The model under review builds one solid part; all positions refer to its coordinate system, in mm. Face numbers are marked on the shaded views. Give positions to 0.01 mm unless a question says otherwise; leave off trailing zeros. Loops run counter-clockwise (first coordinate to the right, second up) from the corner with the lowest first, then second, coordinate; pieces in that order, holes last. Notation, with made-up numbers: M -23.75,84 L 8.25,84 A14 cw 8.25,92 Z; hole C 5,58.25 d4. An arc over 180 degrees is marked long. Return JSON: item names as keys, results as strings. Group by question number.
```python
from build123d import *

# Parameters (mm, degrees)
F0_W     = 85
F0_H     = 19.05
F1_DEPTH = 6.35
F2_R     = 3
F3_R     = 1.535965
F3_R_2   = 4.709265
F4_DEPTH = 25
F5_R     = 1.5
F6_DEPTH = 5


with BuildPart() as f1:
    # F0 (on Front) → F1 (new body)
    with BuildSketch(Plane.XZ):
        Rectangle(F0_W, F0_H)
    extrude(amount=F1_DEPTH)

    # F2
    f2_edges = [f1.edges().sort_by_distance(p)[0] for p in [
        (-42.5, -3.175, 9.525),
        (42.5, -3.175, 9.525),
        (-42.5, -3.175, -9.525),
        (42.5, -3.175, -9.525),
    ]]
    fillet(f2_edges, radius=F2_R)

    # F3 (on face) → F4 (cut)
    with BuildSketch(Plane.XZ.offset(6.35)):
        with Locations((-19.519491, 0)):
            Circle(F3_R)
        with Locations((27.747195, 0)):
            Circle(F3_R_2)
    extrude(amount=-F4_DEPTH, mode=Mode.SUBTRACT)

    # F5 (on face) → F6 (cut)
    with BuildSketch(Plane(origin=(0, 0, -9.525), x_dir=(1, 0, 0), z_dir=(0, 0, -1))):
        with Locations((-21, 3.0625)):
            Circle(F5_R)
        with Locations((21.000085, 3.118848)):
            Circle(F5_R)
    extrude(amount=-F6_DEPTH, mode=Mode.SUBTRACT)


solid = f1.part
```
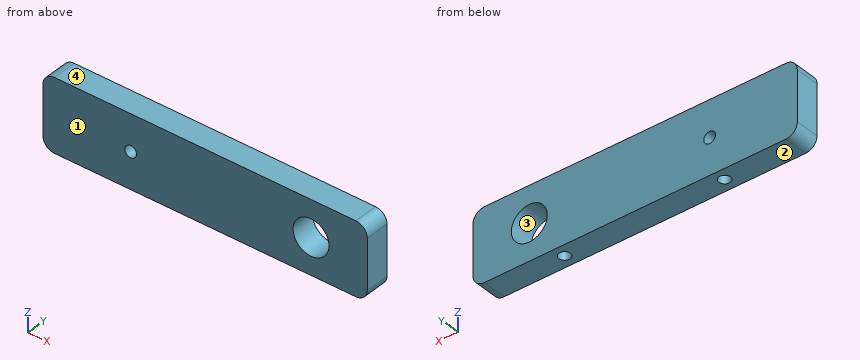
(1) Add section B-B (z = 3.5). Write out the cut boundary in (x, y), and give its area (3 significant figures).
(2) Add section C-C (x = 27). Write out the cut boundary in (y, z) (3 decimals).
(3) Add section A-A (z = 0). Write out the cut boundary in (x, y).
(4) Mouldability with a two-part tool opening along Z and no side actions: class the marked faces 1, 2, 3 and 4 as released by +Z, released by -Z, zero draft, split by the parting line, or undercut.
(5) Add section D-D (z = -8). Write out the cut boundary in (x, y), and give its area (3 significant figures).
(6) For probe 1 along X at (y, z) = (-3.5, 0.5); probe 2 along X at (y, z) = (-3.5, -1); probe 3 along X at (y, z) = (-1.75, -3.5), list the stretches that pass through material, from the lowest coordinate up.
(7) For pin 1 (6 mm diameter, centred on x = -25, z = -3, fed in from +Y); pin 2 (1.5 mm diameter, centred on x = 21.5, y = -3, fed in from -Z) (3 decimals); pin 3 (2.5 mm diameter, centred on x = -19.52, z = 0, fed in from +Y), all flat-tipped, find the tip position at first contact; note any pin that passes through.
Verdict:
{
 "1": {"outline": "M -42.5,-6.35 L 24.6,-6.35 L 24.6,0 L -42.5,0 Z; M 30.9,-6.35 L 42.5,-6.35 L 42.5,0 L 30.9,0 Z", "area": "500 mm²"},
 "2": {"outline": "M -6.35,-9.525 L 0,-9.525 L 0,-4.65 L -6.35,-4.65 Z; M -6.35,4.65 L 0,4.65 L 0,9.525 L -6.35,9.525 Z"},
 "3": {"outline": "M -42.5,-6.35 L -21.06,-6.35 L -21.06,0 L -42.5,0 Z; M -17.98,-6.35 L 23.04,-6.35 L 23.04,0 L -17.98,0 Z; M 32.46,-6.35 L 42.5,-6.35 L 42.5,0 L 32.46,0 Z"},
 "4": {"face 1": "zero draft", "face 2": "released by -Z", "face 3": "undercut", "face 4": "released by +Z"},
 "5": {"outline": "M -42.11,-6.35 L 42.11,-6.35 L 42.11,0 L -42.11,0 Z; hole C -21,-3.06 d3; hole C 21,-3.12 d3", "area": "521 mm²"},
 "6": {"probe 1": "x = -42.5 to -20.97, -18.07 to 23.06, 32.43 to 42.5", "probe 2": "x = -42.5 to -20.69, -18.35 to 23.15, 32.35 to 42.5", "probe 3": "x = -42.5 to 24.6, 30.9 to 42.5"},
 "7": {"pin 1": "stops at y = 0", "pin 2": "stops at z = -4.525", "pin 3": "passes through"}
}
